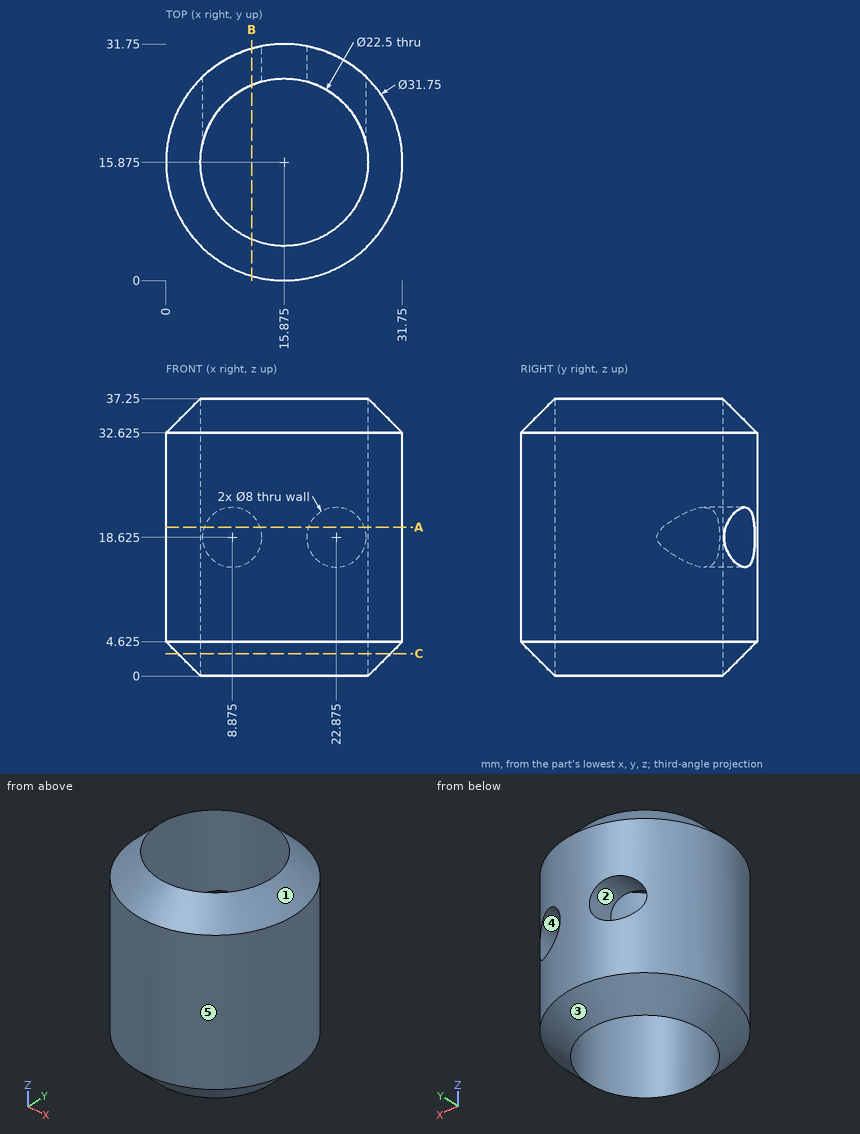
Check sheet for the drawn part. Datum: minimum x, y, z corner. Units: mm. A direction names the side the tool comes from. Give positions to 0.01 mm unless a question says otherwise; leave off trailing zeros. Loops run counter-clockwise (first coordinate to the right, second up) from the corner with the lowest first, then second, coordinate; pieces in that order, holes last.
1) Depth check by flat-ended pin: pin 1 Ø1.5 at (y, z) = (23.5, 31.5) entering from +X; pin 2 Ø6 at (y, z) = (9, 24) entering from -X; pin 3 Ø1.5 at (x, z) = (21, 29) entering from +Y. Enter the tip coordinate at first touch or a pass-through.
2) Set-up check for the marked faces 4 and 5: record each of +Z, -Z, +X, -X, +Y, -Y from which the full face is reachable in a straight line by a thin tool's end or side.
3) Thickness scan on line 1 along Y through (x, z) = (19, 17); line 2 along X through (y, z) = (9.5, 3.5); line 3 along Y through (x, z) = (15.5, 33.5). Record the ranges inside material, lowest first.
4) Sectioned sample at C-C, the plane z = 3. Enter the section's corners in (x, y) (3 decimals), then the cut area to 3 significant figures.
5) Sectioned sample at A-A, the plane z = 20. Enter the section's corners in (x, y) (3 decimals), then the cut area to 3 significant figures.
6) Sectioned sample at B-B, the plane x = 11.5. Count the separate pieces of the cut face and the enclosed holes in it, then the cut area to 3 significant figures.
7) Draft check along Z on the marked faces 1, 2 and 3. Enter one of: pulls with the +Z half, pulls with the -Z half, needs draft (parallel to the pull), parting line crosses it, or undercut.
Answers:
1. pin 1: stops at x = 30.18
1. pin 2: stops at x = 0.48
1. pin 3: stops at y = 31.14
2. face 4: +Y
2. face 5: +Z, -Z
3. line 1: y = 0.31 to 5.07, 26.68 to 31.44
3. line 2: x = 2.57 to 6.61, 25.14 to 29.18
3. line 3: y = 0.88 to 4.63, 27.12 to 30.87
4. outline: circle Ø28.5 at (15.875, 15.875); hole circle Ø22.5 at (15.875, 15.875)
4. area: 240 mm2
5. outline: (5.119, 19.171) - (5.119, 27.551) arc R15.875 ccw (long way) to (26.631, 27.551) - (26.631, 19.171) arc R11.25 cw (long way) to start; (12.631, 26.647) arc R11.25 cw to (19.119, 26.647) - (19.119, 31.415) arc R15.875 ccw to (12.631, 31.415) - close
5. area: 308 mm2
6. separate pieces: 3
6. enclosed holes: 0
6. area: 290 mm2
7. face 1: pulls with the +Z half
7. face 2: undercut
7. face 3: pulls with the -Z half
